Verification items for this drawing (mm, ordinates from the low corner). A direction names the side the tool comes from. Round coordinates to 2 decimals unless told otherwise and drop trailing zeros. Order: outer loops, then holes, each group sorted by start corner. A loop starts at its lowest first (then second) coordinate and runs counter-clockwise, first axis right, second up. Notation, with made-up numbers: (52.25, 25.25) -> (97.25, 25.25) arc R31 ccw to (97.25, 52.25) -> close; hole circle Ø6 at (74, 11.25). An arc over 180 degrees is marked (long way). Answer in a Markdown table with one row per item.
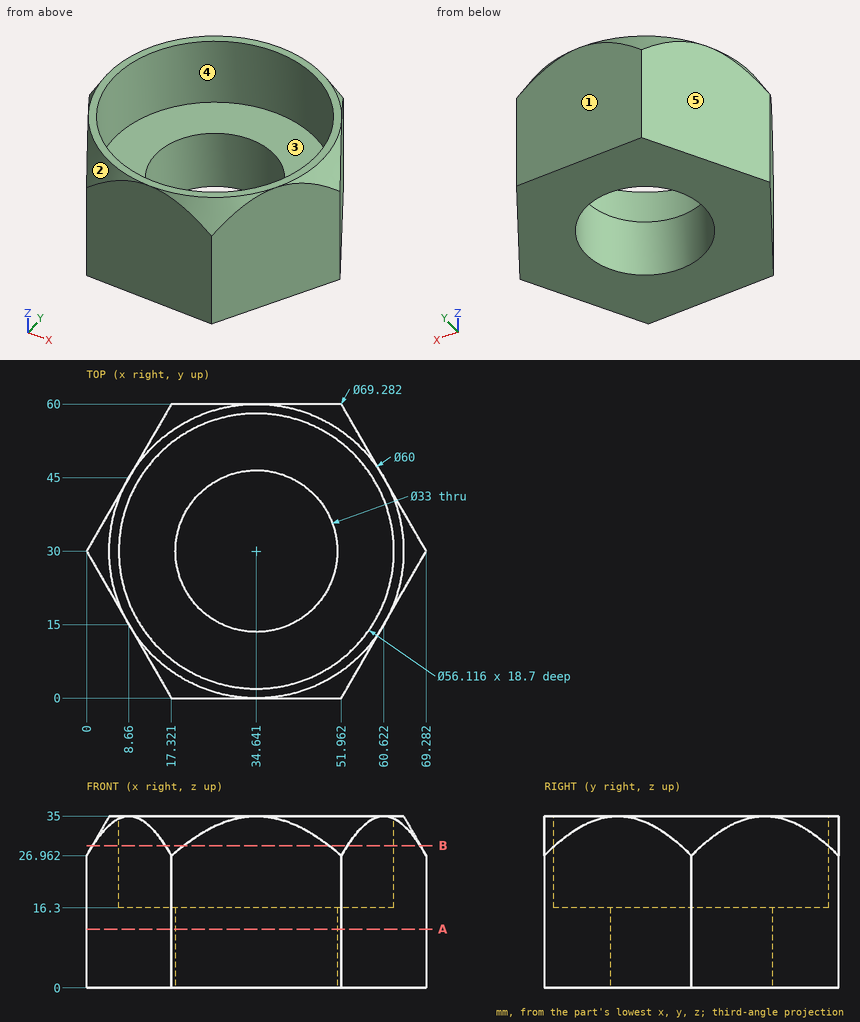
Item 1: Mould release check, pull along X, two halves, no side actions. Record for the marked faces 1, 2 and 3: pulls with the +X half, pulls with the -X half, needs draft (parallel to the pull), parting line crosses it, or undercut.
Result sheet:
| item | result |
|---|---|
| face 1 | needs draft |
| face 2 | pulls with the -X half |
| face 3 | undercut |
Item 2: Set-up check for the marked faces 4 and 5: record each of +Z, -Z, +X, -X, +Y, -Y from which the full face is reachable in a straight line by a thin tool's end or side.
Result sheet:
| item | result |
|---|---|
| face 4 | +Z |
| face 5 | +Z, -Z, -X, +Y |
Item 3: Cross-section at B-B (z = 29). Record the boundary of the cut face in (x, y) (1 decimal).
Result sheet:
| item | result |
|---|---|
| outline | (1.2, 27.8) -> (16.1, 2.2) arc R33.5 ccw to (19.8, 0) -> (49.5, 0) arc R33.5 ccw to (53.2, 2.2) -> (68, 27.8) arc R33.5 ccw to (68, 32.2) -> (53.2, 57.8) arc R33.5 ccw to (49.5, 60) -> (19.8, 60) arc R33.5 ccw to (16.1, 57.8) -> (1.2, 32.2) arc R33.5 ccw to start; hole circle Ø56.1 at (34.6, 30) |
Item 4: Depth check by flat-ended pin: P1, Ø4, axis at y = 51.5, z = 12, coming from the +X side (1 decimal); P2, Ø4, axis at x = 40.5, y = 13.5, coming from the +Z side; P3, Ø5, axis at y = 33.5, z = 8, coming from the +X side (1 decimal). Enter the tip coordinate at first touch or a pass-through.
Result sheet:
| item | result |
|---|---|
| P1 | stops at x = 58 |
| P2 | stops at z = 16.3 |
| P3 | stops at x = 68.7 |
Item 5: Scan lines: line 1 (Z direction, x = 10.5, y = 22.5); line 2 (Y direction, x = 60.5, z = 32.5) (1 decimal); line 3 (Y direction, x = 23.5, z = 21). Record each from-to range of solid material in increasing order. Write a range as [from, to].
Result sheet:
| item | result |
|---|---|
| line 1 | z = [0, 16.3] |
| line 2 | y = [14.8, 19.1], [40.9, 45.2] |
| line 3 | y = [0, 4.25], [55.75, 60] |
Item 6: Cross-section at A-A (z = 12). Record the boundary of the cut face in (x, y).
Result sheet:
| item | result |
|---|---|
| outline | (0, 30) -> (17.32, 0) -> (51.96, 0) -> (69.28, 30) -> (51.96, 60) -> (17.32, 60) -> close; hole circle Ø33 at (34.64, 30) |
